Could you check a few things on this model? Use its own coordinates, in mm. Face numbers are marked on the shaded views. Coordinates: 2 decimals unless noted, no trailing zeros. Loops run counter-clockwise (first coordinate to the right, second up) from the corner with the lowest first, then second, coordinate; pieces in that order, holes last. Notation, with made-up numbers: (19, 87) -> (71, 87) arc R13 cw to (71, 103) -> close; hole circle Ø5 at (10.5, -12.75). An arc over 180 degrees is marked (long way). One line per question, with ' | ' between items.
Autodesk Inventor part; units mm, degrees
ref_plane "YZ Plane" through (0, 0, 0) normal (1, 0, 0) x (0, 1, 0)
ref_plane "XZ Plane" through (0, 0, 0) normal (0, 1, 0) x (-1, 0, 0)
ref_plane "XY Plane" through (0, 0, 0) normal (0, 0, 1) x (1, 0, 0)
sketch "Esboço1" plane through (0, 0, 0) normal (0, 1, 0) x (-1, 0, 0)
  circle A0 centre (0, 0) radius 6
  dimension "d0" = 12
extrude "Extrusão1" add sketch "Esboço1" along normal blind 9.5
sketch "Esboço2" plane through (0, 9.5, 0) normal (0, 1, 0) x (1, 0, 0)
  line L0 (0, 0) -> (0, 3.8)
  circle A0 centre (0, 3.8) radius 0.3
  dimension "d3" = 3.8
  dimension "d4" = 0.6
extrude "Extrusão2" add sketch "Esboço2" along normal blind 5
sketch "Esboço3" plane through (0, 9.5, 0) normal (0, 1, 0) x (1, 0, 0)
  circle A0 centre (0, 3.8) radius 0.3
  line L0 (0, 3.8) -> (0, -3.8)
  circle A1 centre (0, -3.8) radius 0.3
  point P0 (0, 0)
  dimension "d7" = 7.6
extrude "Extrusão3" add sketch "Esboço3" along normal blind 6.2 contours A1
sketch "Esboço4" plane through (0, 9.5, 0) normal (0, 1, 0) x (1, 0, 0)
  line L0 (-0.9551, -5.4164) -> (-1.0419, -5.9088)
  circle A0 centre (0, 0) radius 6
  line L1 (0, 0) -> (6, 0) construction
  line L2 (0.9551, -5.4164) -> (1.0419, -5.9088)
  arc A1 (-1.0419, -5.9088) -> (1.0419, -5.9088) centre (0, 0) ccw
  line L3 (0, -6) -> (0, -5.5)
  line L4 (1.0419, -5.9088) -> (0.9551, -5.4164)
  line L5 (-1.0419, -5.9088) -> (-0.9551, -5.4164)
  arc A2 (-0.9551, -5.4164) -> (0.9551, -5.4164) centre (0, 0) ccw
  line L6 (5.1683, 1.8811) -> (5.6382, 2.0521)
  line L7 (4.2132, 3.5353) -> (4.5963, 3.8567)
  arc A3 (5.6382, 2.0521) -> (4.5963, 3.8567) centre (0, 0) ccw
  line L8 (5.1962, 3) -> (4.7631, 2.75)
  line L9 (4.5963, 3.8567) -> (4.2132, 3.5353)
  line L10 (5.6382, 2.0521) -> (5.1683, 1.8811)
  arc A4 (5.1683, 1.8811) -> (4.2132, 3.5353) centre (0, 0) ccw
  line L11 (-4.2132, 3.5353) -> (-4.5963, 3.8567)
  line L12 (-5.1683, 1.8811) -> (-5.6382, 2.0521)
  arc A5 (-4.5963, 3.8567) -> (-5.6382, 2.0521) centre (0, 0) ccw
  line L13 (-5.1962, 3) -> (-4.7631, 2.75)
  line L14 (-5.6382, 2.0521) -> (-5.1683, 1.8811)
  line L15 (-4.5963, 3.8567) -> (-4.2132, 3.5353)
  arc A6 (-4.2132, 3.5353) -> (-5.1683, 1.8811) centre (0, 0) ccw
  dimension "d10" = 100
  dimension "d11" = 0.5
  dimension "d12" = 0.5
  dimension "d13" = 0.5
  dimension "d16" = 360
extrude "Extrusão4" add sketch "Esboço4" along normal blind 0.5 contours A2 L3 A0 L0 | A2 L2 A0 L3 | A0 L13 A6 L12 | A0 L11 A6 L13 | A0 L8 A4 L7 | L6 A4 L8 A0
sketch "Esboço5" plane through (0, 0, 0) normal (0, -1, 0) x (1, 0, 0)
  circle A0 centre (0, 0) radius 1.1
  dimension "d20" = 2.2
extrude "Extrusão5" cut sketch "Esboço5" against normal blind 2
sketch "Esboço6" plane through (0, 0, 0) normal (0, -1, 0) x (1, 0, 0)
  circle A0 centre (0, 0) radius 6
  line L0 (0, 6) -> (0, 4.5)
  circle A1 centre (0, 4.5) radius 1
  circle A2 centre (0, 4.5) radius 0.75
  line L1 (0, 5.25) -> (0, 5.15)
  line L2 (0, 5.15) -> (-0.2, 5.15)
  line L3 (-0.2, 5.15) -> (-0.2, 4.7)
  line L4 (-0.2, 4.7) -> (-0.65, 4.7)
  line L5 (-0.65, 4.7) -> (-0.65, 4.3)
  line L6 (-0.65, 4.3) -> (-0.2, 4.3)
  line L7 (-0.2, 4.3) -> (-0.2, 3.85)
  line L8 (-0.2, 3.85) -> (0.2, 3.85)
  line L9 (0.2, 3.85) -> (0.2, 4.3)
  line L10 (0.2, 4.3) -> (0.65, 4.3)
  line L11 (0.65, 4.3) -> (0.65, 4.7)
  line L12 (0.65, 4.7) -> (0.2, 4.7)
  line L13 (0, 5.15) -> (0.2, 5.15)
  line L14 (0.2, 5.15) -> (0.2, 4.7)
  dimension "d25" = 1.5
  dimension "d23" = 1.5
  dimension "d24" = 2
  dimension "d26" = 0.1
  dimension "d27" = 0.2
  dimension "d28" = 0.45
  dimension "d29" = 0.45
  dimension "d30" = 0.4
  dimension "d31" = 0.45
  dimension "d32" = 0.4
  dimension "d33" = 0.45
  dimension "d34" = 0.2
extrude "Extrusão6" cut sketch "Esboço6" against normal blind 0.01 contours L13 L14 L12 L11 L10 L9 L8 L7 L6 L5 L4 L3 L2 | A1
sketch "Esboço7" plane through (0, 9.5, 0) normal (0, 1, 0) x (1, 0, 0)
  circle A0 centre (0, 0) radius 1.1
  circle A1 centre (0, 0) radius 6
  circle A2 centre (0, 0) radius 5.5
extrude "Extrusão7" add sketch "Esboço7" along normal blind 0.1 contours A1
properties part number "Buzzer 5v" material "Plástico PBT"
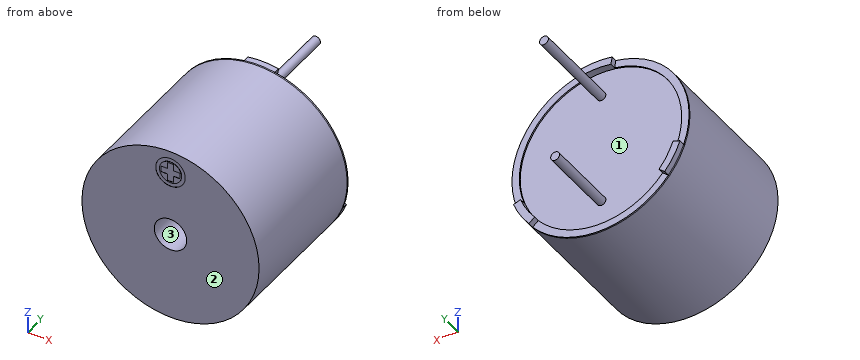
Q1. For pin 1 (4 mm diameter, centred on x = 3, z = 4, fed in from +Y); pin 2 (1.5 mm diameter, centred on x = -2, y = 13, fed in from -Z); pin 3 (0.7 mm diameter, centred on x = -5, z = -3, fed in from +Y); pin 4 (3.5 mm diameter, centred on x = 1.5, z = -0.5, fed in from +Y), each with a flat end and sliding along its axis, tell me the tip position at first contact or that it passes through.
Values follow:
pin 1: stops at y = 9.6 | pin 2: passes through | pin 3: stops at y = 10 | pin 4: stops at y = 9.5
Q2. Please list where these lines run through material, in increasing order: L1, parallel to Z at x = 0, y = 0.95; L2, parallel to Y at x = -4.75, z = -1; L3, parallel to Z at x = 1.25, y = 7. Write a range as [from, to].
Values follow:
L1: z = [-6, -1.1], [1.1, 6] | L2: y = [0, 9.5] | L3: z = [-5.87, 5.87]
Q3. Imagine slicing it at C-C on z = -2.25. Write out the boundary of the cut face in (x, y).
Values follow:
outline: (-5.56, 0) -> (5.56, 0) -> (5.56, 10) -> (5.02, 10) -> (5.02, 9.5) -> (-5.02, 9.5) -> (-5.02, 10) -> (-5.56, 10) -> close
Q4. Imagine slicing it at B-B on y = 1.25. Write out the boundary of the cut face in (x, z).
Values follow:
outline: circle Ø12 at (0, 0); hole circle Ø2.2 at (0, 0)
Q5. Imagine slicing it at D-D on x = -3.5. Write out the boundary of the cut face in (y, z).
Values follow:
outline: (0, -4.87) -> (9.6, -4.87) -> (9.6, -4.24) -> (9.5, -4.24) -> (9.5, 4.24) -> (9.6, 4.24) -> (9.6, 4.87) -> (0, 4.87) -> close
Q6. We'd pull the mould along X, two halves only. Please class the marked faces 1, 2 and 3: released by +X, released by -X, zero draft, split by the parting line, or undercut.
Values follow:
face 1: undercut | face 2: zero draft | face 3: undercut
